Design review of the part built by this model. Coordinates are the model's own, in mm. A direction names the side the tool comes from. Coordinates: 2 decimals unless noted, no trailing zeros. Loops run counter-clockwise (first coordinate to the right, second up) from the corner with the lowest first, then second, coordinate; pieces in that order, holes last. Notation, with made-up numbers: (-3.5, -27) - (2.5, -27) arc R20 cw to (2.5, -4) - close; hole circle Ø3 at (84.25, 43). An arc over 180 degrees is marked (long way). Answer in a Markdown table with one row per item. Add a question column.
(1) We need section A-A, the plane x = 43.5. Write out the cut boundary in (y, z), plus the area to 3 significant figures.
(2) We need section B-B, the plane z = -32.5. Write out the cut boundary in (x, y), plus the area to 3 significant figures.
(3) For faces 4 (the face through (48, 3, -20.601)), 5 (the face through (11.64, 3.33, -29.2)), 6 (the face through (31.528, 3.818, -4.151)), list the 3-axis set-ups (+Z, -Z, +X, -X, +Y, -Y) from which the entire face can be reached by the end or side of a thin tool; tool diameter is ignored.
(4) The part is to be moulded in two halves that separate along X. For faces 1 (the face through (24, 2.6, -20)), 2 (the face through (36.64, 3.33, -26.71)), 3 (the face through (66.08, 1, -1)), say which applies: released by +X, released by -X, zero draft, split by the parting line, or undercut.
(5) Clearance check with flat-ended pins moving along their axes: pin 1 (5 mm diameter, centred on x = 7, z = -21, fed in from +Y); pin 2 (3.5 mm diameter, centred on x = 66.35, z = -8, fed in from +Y); pin 3 (12 mm diameter, centred on x = 33.5, z = -14, fed in from +Y); pin 4 (1.5 mm diameter, centred on y = 4, z = -36, fed in from -X). State where each tip first meets the part, or that it passes through.
(6) We need section C-C, the plane x = 53. Write out the cut boundary in (y, z), plus the area to 3 significant figures.
(7) To check wall thickness, follow L1, parallel to Z at x = 43, y = 3.25; L2, parallel to X at y = 0.95, z = -36; L3, parallel to Z at x = 66.35, y = 0.8. State the ranges of each line that lie inside material, in increasing order. Write a range as [from, to].
from build123d import *

# Parameters (mm, degrees)
SALIENTE_EXTRUIR1_DEPTH = 1.6
CHAFL_N1_SIZE           = 2.6
CROQUIS2_R              = 1.5
CORTAR_EXTRUIR1_DEPTH   = 87.926822673
CROQUIS3_W              = 35.565034919
CROQUIS3_H              = 8.613377017
SALIENTE_EXTRUIR2_DEPTH = 3
CROQUIS4_R              = 3.336672647
CROQUIS4_R_2            = 3.426556793
SALIENTE_EXTRUIR3_DEPTH = 5
CROQUIS5_W              = 6.263410385
CROQUIS5_H              = 6.323061912
CROQUIS5_W_2            = 3.698394703
CROQUIS5_H_2            = 4.23525845
CROQUIS5_W_3            = 2.624667209
CROQUIS5_H_3            = 4.444038797
CROQUIS5_W_4            = 2.684318736
CROQUIS5_H_4            = 1.371985132
CROQUIS5_W_5            = 4.831773725
CROQUIS5_H_5            = 5.010728307
SALIENTE_EXTRUIR4_DEPTH = 1
SALIENTE_EXTRUIR5_DEPTH = 4
REDONDEO1_R             = 0.5


with BuildPart() as part:
    # Croquis1 → Saliente-Extruir1 (new body)
    with BuildSketch(Plane(origin=(0, 0, 0), x_dir=(1, 0, 0), z_dir=(0, 1, 0))):
        Polygon((0, 53.3), (66.08, 53.3), (66.08, 39.738845798), (68.65, 39.738845798), (68.65, 2.138845798), (66.08, 2.138845798), (66.08, 0), (0, 0), align=None)
    extrude(amount=SALIENTE_EXTRUIR1_DEPTH)

    # Chaflán1
    # the kernel refuses this chamfer: 2.6 mm, written as the material it takes off along each edge
    with BuildSketch(Plane(origin=(68.65, -6.686375769, -39.738845798), x_dir=(-0.9996219169112966, 0, -0.027495876610585446), z_dir=(0, 1, 0))) as chafl_n1_piece_1_section:
        Polygon((CHAFL_N1_SIZE * 0.999621916911, CHAFL_N1_SIZE * 0.0274958766106), (-CHAFL_N1_SIZE * 0.0274958766106, CHAFL_N1_SIZE * 0.999621916911), (0, 0), align=None)
    chafl_n1_piece_1 = extrude(amount=14.972751537, mode=Mode.PRIVATE)
    chafl_n1_piece_1 = split(chafl_n1_piece_1, bisect_by=Plane(origin=(66.08, 0.8, -38.878812764), z_dir=(1, 0, 0)), keep=Keep.TOP, mode=Mode.PRIVATE)
    add(chafl_n1_piece_1, mode=Mode.SUBTRACT)
    with BuildSketch(Plane(origin=(68.65, -6.686375769, -2.138845798), x_dir=(0.027495876610585345, 0, -0.9996219169112966), z_dir=(0, 1, 0))) as chafl_n1_piece_2_section:
        Polygon((CHAFL_N1_SIZE * 0.999621916911, CHAFL_N1_SIZE * 0.0274958766106), (-CHAFL_N1_SIZE * 0.0274958766106, CHAFL_N1_SIZE * 0.999621916911), (0, 0), align=None)
    chafl_n1_piece_2 = extrude(amount=14.972751537, mode=Mode.PRIVATE)
    chafl_n1_piece_2 = split(chafl_n1_piece_2, bisect_by=Plane(origin=(66.08, 0.8, -2.998878832), z_dir=(1, 0, 0)), keep=Keep.TOP, mode=Mode.PRIVATE)
    add(chafl_n1_piece_2, mode=Mode.SUBTRACT)
    with BuildSketch(Plane(origin=(66.08, -6.686375769, -53.3), x_dir=(-0.9996219169112966, 0, -0.027495876610585373), z_dir=(0, 1, 0))) as chafl_n1_piece_3:
        Polygon((CHAFL_N1_SIZE * 0.999621916911, CHAFL_N1_SIZE * 0.0274958766106), (-CHAFL_N1_SIZE * 0.0274958766106, CHAFL_N1_SIZE * 0.999621916911), (0, 0), align=None)
    extrude(amount=14.972751537, mode=Mode.SUBTRACT)

    # Croquis2 → Cortar-Extruir1 (cut, through all)
    with BuildSketch(Plane(origin=(0, 1.6, 0), x_dir=(1, 0, 0), z_dir=(0, 1, 0))):
        with Locations(Location((15.5, 51, 0), (0, 0, 270))):
            Circle(CROQUIS2_R)
        with Locations(Location((66.35, 36, 0), (0, 0, 270))):
            Circle(CROQUIS2_R)
        with Locations(Location((66.35, 8, 0), (0, 0, 270))):
            Circle(CROQUIS2_R)
        with Locations(Location((14, 2.3, 0), (0, 0, 270))):
            Circle(CROQUIS2_R)
    extrude(amount=-CORTAR_EXTRUIR1_DEPTH, mode=Mode.SUBTRACT)

    # Croquis3 → Saliente-Extruir2 (add)
    with BuildSketch(Plane(origin=(0, 1.6, 0), x_dir=(1, 0, 0), z_dir=(0, 1, 0))):
        with Locations((47.771511194, 16.294435422)):
            Rectangle(CROQUIS3_W, CROQUIS3_H)
    extrude(amount=SALIENTE_EXTRUIR2_DEPTH)

    # Croquis4 → Saliente-Extruir3 (add)
    with BuildSketch(Plane(origin=(0, 1.6, 0), x_dir=(1, 0, 0), z_dir=(0, 1, 0))):
        with Locations(Location((28.27044436, 4.874550457, 0), (0, 0, 90))):
            Circle(CROQUIS4_R)
        with Locations(Location((19.960106187, 4.874550457, 0), (0, 0, 90))):
            Circle(CROQUIS4_R_2)
    extrude(amount=SALIENTE_EXTRUIR3_DEPTH)

    # Croquis5 → Saliente-Extruir4 (add)
    with BuildSketch(Plane(origin=(0, 1.6, 0), x_dir=(1, 0, 0), z_dir=(0, 1, 0))):
        with Locations((5.120871528, 17.658331847)):
            Rectangle(CROQUIS5_W, CROQUIS5_H)
        with Locations((23.642670808, 19.775961072)):
            Rectangle(CROQUIS5_W_2, CROQUIS5_H_2)
        with Locations((14.87389627, 17.553941673)):
            Rectangle(CROQUIS5_W_3, CROQUIS5_H_3)
        with Locations((24.149708791, 12.617777775)):
            Rectangle(CROQUIS5_W_4, CROQUIS5_H_4)
        with Locations((19.377586593, 38.417063407)):
            Rectangle(CROQUIS5_W_5, CROQUIS5_H_5)
    extrude(amount=SALIENTE_EXTRUIR4_DEPTH)

    # Croquis6 → Saliente-Extruir5 (add)
    with BuildSketch(Plane(origin=(0, 1.6, 0), x_dir=(1, 0, 0), z_dir=(0, 1, 0))):
        with BuildLine():
            Line((14.144691977, 31.757239244), (20.991330498, 31.757239244))
            ThreePointArc((20.991330498, 31.757239244), (23.496200875, 29.252368867), (20.991330498, 26.74749849))
            Line((20.991330498, 26.74749849), (14.144691977, 26.74749849))
            ThreePointArc((14.144691977, 26.74749849), (11.6398216, 29.252368867), (14.144691977, 31.757239244))
        make_face()
        with BuildLine():
            Line((38.431163378, 28.540921146), (45.590129983, 28.540921146))
            ThreePointArc((45.590129983, 28.540921146), (47.383552638, 26.74749849), (45.590129983, 24.954075835))
            Line((45.590129983, 24.954075835), (38.431163378, 24.954075835))
            ThreePointArc((38.431163378, 24.954075835), (36.637740722, 26.74749849), (38.431163378, 28.540921146))
        make_face()
    extrude(amount=SALIENTE_EXTRUIR5_DEPTH)

    # Redondeo1
    redondeo1_edges = [part.edges().sort_by_distance(p)[0] for p in [
        (11.6398216, 5.6, -29.252368867),
        (17.568011237, 5.6, -26.74749849),
        (23.496200875, 5.6, -29.252368867),
        (17.568011237, 5.6, -31.757239244),
        (36.637740722, 5.6, -26.74749849),
        (42.01064668, 5.6, -24.954075835),
        (47.383552638, 5.6, -26.74749849),
        (42.01064668, 5.6, -28.540921146),
        (28.27044436, 6.6, -1.53787781),
        (19.960106187, 6.6, -1.447993664),
    ]]
    fillet(redondeo1_edges, radius=REDONDEO1_R)


solid = part.part
Responses:
| question | item | result |
|---|---|---|
| 1 | outline | (0, -53.3) - (1.6, -53.3) - (1.6, -28.54) - (5.1, -28.54) arc R0.5 ccw to (5.6, -28.04) - (5.6, -25.45) arc R0.5 ccw to (5.1, -24.95) - (1.6, -24.95) - (1.6, -20.6) - (4.6, -20.6) - (4.6, -11.99) - (1.6, -11.99) - (1.6, 0) - (0, 0) - close |
| 1 | area | 125 mm2 |
| 2 | outline | (0, 0) - (68.65, 0) - (68.65, 1.6) - (0, 1.6) - close |
| 2 | area | 110 mm2 |
| 3 | face 4 | +X, +Y |
| 3 | face 5 | -X, +Y |
| 3 | face 6 | +Y |
| 4 | face 1 | zero draft |
| 4 | face 2 | undercut |
| 4 | face 3 | released by +X |
| 5 | pin 1 | stops at y = 2.6 |
| 5 | pin 2 | stops at y = 1.6 |
| 5 | pin 3 | stops at y = 4.6 |
| 5 | pin 4 | passes through |
| 6 | outline | (0, -53.3) - (1.6, -53.3) - (1.6, -20.6) - (4.6, -20.6) - (4.6, -11.99) - (1.6, -11.99) - (1.6, 0) - (0, 0) - close |
| 6 | area | 111 mm2 |
| 7 | L1 | z = [-28.54, -24.95], [-20.6, -11.99] |
| 7 | L2 | x = [0, 64.85], [67.85, 68.65] |
| 7 | L3 | z = [-39.44, -37.5], [-34.5, -9.5], [-6.5, -2.44] |
